```python
from build123d import *

# Parameters (mm, degrees)
SKETCH_1_W          = 95
SKETCH_1_H          = 75
EXTRUDE_1_DEPTH     = 5
HOLE_WIZARD_M5_1_D  = 5.3
CUT_EXTRUDE_2_DEPTH = 6
CUT_EXTRUDE_3_REACH = 7
SKETCH_4_R          = 8
SKETCH_8_W          = 95
SKETCH_8_H          = 5
EXTRUDE_2_DEPTH     = 40
CUT_EXTRUDE_4_REACH = 7
SKETCH_9_R          = 9.6
CUT_EXTRUDE_5_REACH = 7
SKETCH_10_R         = 4.1
CUT_EXTRUDE_6_REACH = 7
SKETCH_11_R         = 6.5
CHAMFER_2_SIZE      = 10


with BuildPart() as part:
    # 草圖1 → 填料-伸長1 (new body)
    with BuildSketch(Plane.XY):
        Rectangle(SKETCH_1_W, SKETCH_1_H)
    extrude(amount=EXTRUDE_1_DEPTH)

    # M5 餘隙孔1 (through all)
    with Locations(Plane.XY.offset(5)):
        with Locations((27.5, 27.5), (7.5, 7.5), (7.5, 27.5), (27.5, 7.5)):
            Hole(HOLE_WIZARD_M5_1_D / 2)

    # 草圖6 → 除料-伸長2 (cut, through all)
    with BuildSketch(Plane.XY.offset(5)):
        with BuildLine():
            Line((-37.7, -6.5), (-37.7, 11.5))
            ThreePointArc((-37.7, 11.5), (-26.5, 22.7), (-15.3, 11.5))
            Line((-15.3, 11.5), (-15.3, -6.5))
            ThreePointArc((-15.3, -6.5), (-26.5, -17.7), (-37.7, -6.5))
        make_face()
        with BuildLine():
            Line((-40.4, 27), (-40.4, 9))
            ThreePointArc((-40.4, 9), (-42, 7.4), (-43.6, 9))
            Line((-43.6, 9), (-43.6, 27))
            ThreePointArc((-43.6, 27), (-42, 28.6), (-40.4, 27))
        make_face()
        with BuildLine():
            Line((-9.4, 27), (-9.4, 9))
            ThreePointArc((-9.4, 9), (-11, 7.4), (-12.6, 9))
            Line((-12.6, 9), (-12.6, 27))
            ThreePointArc((-12.6, 27), (-11, 28.6), (-9.4, 27))
        make_face()
        with BuildLine():
            Line((-9.4, -4), (-9.4, -22))
            ThreePointArc((-9.4, -22), (-11, -23.6), (-12.6, -22))
            Line((-12.6, -22), (-12.6, -4))
            ThreePointArc((-12.6, -4), (-11, -2.4), (-9.4, -4))
        make_face()
        with BuildLine():
            Line((-40.4, -4), (-40.4, -22))
            ThreePointArc((-40.4, -22), (-42, -23.6), (-43.6, -22))
            Line((-43.6, -22), (-43.6, -4))
            ThreePointArc((-43.6, -4), (-42, -2.4), (-40.4, -4))
        make_face()
    extrude(amount=-CUT_EXTRUDE_2_DEPTH, mode=Mode.SUBTRACT)

    # 草圖4 → 除料-伸長3 (cut, up to next)
    with BuildSketch(Plane.XY.offset(5), mode=Mode.PRIVATE) as cut_extrude_3_sk1:
        with Locations((35.5, -24)):
            Circle(SKETCH_4_R)
    cut_extrude_3_tool1 = extrude(cut_extrude_3_sk1.sketch, amount=-CUT_EXTRUDE_3_REACH, mode=Mode.PRIVATE) & part.part
    add(cut_extrude_3_tool1.solids().sort_by_distance((35.5, -24, 5))[0], mode=Mode.SUBTRACT)

    # 草圖8 → 填料-伸長2 (add)
    with BuildSketch(Plane(origin=(0, 37.5, 0), x_dir=(1, 0, 0), z_dir=(0, 1, 0))):
        with Locations((0, -2.5)):
            Rectangle(SKETCH_8_W, SKETCH_8_H)
    extrude(amount=EXTRUDE_2_DEPTH)

    # 草圖9 → 除料-伸長4 (cut, up to next)
    with BuildSketch(Plane.XY.offset(5), mode=Mode.PRIVATE) as cut_extrude_4_sk1:
        with Locations((27.5, 57.5)):
            Circle(SKETCH_9_R)
    cut_extrude_4_tool1 = extrude(cut_extrude_4_sk1.sketch, amount=-CUT_EXTRUDE_4_REACH, mode=Mode.PRIVATE) & part.part
    add(cut_extrude_4_tool1.solids().sort_by_distance((27.5, 57.5, 5))[0], mode=Mode.SUBTRACT)

    # 草圖10 → 除料-伸長5 (cut, up to next)
    with BuildSketch(Plane.XY.offset(5), mode=Mode.PRIVATE) as cut_extrude_5_sk1:
        with Locations((0, 65)):
            Circle(SKETCH_10_R)
    cut_extrude_5_tool1 = extrude(cut_extrude_5_sk1.sketch, amount=-CUT_EXTRUDE_5_REACH, mode=Mode.PRIVATE) & part.part
    add(cut_extrude_5_tool1.solids().sort_by_distance((0, 65, 5))[0], mode=Mode.SUBTRACT)
    # 草圖10 → 除料-伸長5 (cut, up to next)
    with BuildSketch(Plane.XY.offset(5), mode=Mode.PRIVATE) as cut_extrude_5_sk2:
        with Locations((0, 50)):
            Circle(SKETCH_10_R)
    cut_extrude_5_tool2 = extrude(cut_extrude_5_sk2.sketch, amount=-CUT_EXTRUDE_5_REACH, mode=Mode.PRIVATE) & part.part
    add(cut_extrude_5_tool2.solids().sort_by_distance((0, 50, 5))[0], mode=Mode.SUBTRACT)

    # 草圖11 → 除料-伸長6 (cut, up to next)
    with BuildSketch(Plane.XY.offset(5), mode=Mode.PRIVATE) as cut_extrude_6_sk1:
        with Locations((-27.5, 57.5)):
            Circle(SKETCH_11_R)
    cut_extrude_6_tool1 = extrude(cut_extrude_6_sk1.sketch, amount=-CUT_EXTRUDE_6_REACH, mode=Mode.PRIVATE) & part.part
    add(cut_extrude_6_tool1.solids().sort_by_distance((-27.5, 57.5, 5))[0], mode=Mode.SUBTRACT)

    # 導角2
    chamfer_2_edges = [part.edges().sort_by_distance(p)[0] for p in [
        (47.5, 77.5, 2.5),
        (-47.5, 77.5, 2.5),
        (47.5, -37.5, 2.5),
        (-47.5, -37.5, 2.5),
    ]]
    chamfer(chamfer_2_edges, length=CHAMFER_2_SIZE)


solid = part.part
```
Can you work these out from the model? Positions are in its coordinate system, mm. A direction names the side the tool comes from. Coordinates: 2 decimals unless noted, no trailing zeros. Order: outer loops, then holes, each group sorted by start corner. A loop starts at its lowest first (then second) coordinate and runs counter-clockwise, first axis right, second up.
1. If we section it at C-C (z = 2.85): Give the number of separate pieces and of enclosed holes in the cut face, then the cut area to 3 significant figures.
2. I need wall thicknesses on line 1 (Y direction, x = 7.5, z = 1.7); line 2 (Y direction, x = 0, z = 1.4); line 3 (X direction, y = -2, z = 3.25). Which ranges of each line are inside material? Lowest first, please.
3. If we section it at A-A (y = 21): Please give me the cut outline in (x, z), then the cut area to 3 significant figures.
4. Thinking about a two-plate mould opening in X: for faces 3 (the face through (-42, -33, 2)), 4 (the face through (-9.4, -13, 3)), 5 (the face through (-1, 19, 5)), which applies, +X half, -X half, draft (parallel to the pull), parting line (faces both ways), or undercut?
5. If we section it at D-D (y = 52.5): Please give me the cut outline in (x, z).
6. If we section it at B-B (x = 35.5): Please give me the cut outline in (y, z), then the cut area to 3 significant figures.
7. For faces 1 (the face through (-43.6, -13, 3)), 2 (the face through (-1, -37.5, 2)), which set-ups out of +Z, -Z, +X, -X, +Y, -Y let a thin tool reach every point of the face, with its end or its side?
Entries:
1. separate pieces: 1
1. enclosed holes: 14
1. area: 8,850 mm2
2. line 1: y = -37.5 to 4.85, 10.15 to 24.85, 30.15 to 77.5
2. line 2: y = -37.5 to 45.9, 54.1 to 60.9, 69.1 to 77.5
2. line 3: x = -47.5 to -37.7, -15.3 to 47.5
3. outline: (-47.5, 0) - (-43.6, 0) - (-43.6, 5) - (-47.5, 5) - close; (-40.4, 0) - (-32.43, 0) - (-32.43, 5) - (-40.4, 5) - close; (-20.57, 0) - (-12.6, 0) - (-12.6, 5) - (-20.57, 5) - close; (-9.4, 0) - (47.5, 0) - (47.5, 5) - (-9.4, 5) - close
3. area: 384 mm2
4. face 3: -X half
4. face 4: undercut
4. face 5: draft
5. outline: (-47.5, 0) - (-31.65, 0) - (-31.65, 5) - (-47.5, 5) - close; (-23.35, 0) - (-3.25, 0) - (-3.25, 5) - (-23.35, 5) - close; (3.25, 0) - (19.3, 0) - (19.3, 5) - (3.25, 5) - close; (35.7, 0) - (47.5, 0) - (47.5, 5) - (35.7, 5) - close
6. outline: (-37.5, 0) - (-32, 0) - (-32, 5) - (-37.5, 5) - close; (-16, 0) - (52.19, 0) - (52.19, 5) - (-16, 5) - close; (62.81, 0) - (77.5, 0) - (77.5, 5) - (62.81, 5) - close
6. area: 442 mm2
7. face 1: +Z, -Z
7. face 2: +Z, -Z, +X, -X, -Y
